```python
from build123d import *

# Parameters (mm, degrees)
SKETCH1_R           = 12.74408056
SKETCH1_R_2         = 4.1275
BOSS_EXTRUDE1_DEPTH = 6.35
SKETCH2_R           = 1.8415
CUT_EXTRUDE1_DEPTH  = 177.753707175


with BuildPart() as part:
    # Sketch1 → Boss-Extrude1 (new body)
    with BuildSketch(Plane(origin=(0, 0, 0), x_dir=(1, 0, 0), z_dir=(0, 1, 0))):
        with BuildLine():
            Line((0, -15.24), (158.75, -15.24))
            ThreePointArc((158.75, -15.24), (173.99, 0), (158.75, 15.24))
            Line((158.75, 15.24), (0, 15.24))
            ThreePointArc((0, 15.24), (-15.24, 0), (0, -15.24))
        make_face()
        with Locations(Location((0, 0, 0), (0, 0, 270))):
            Circle(SKETCH1_R, mode=Mode.SUBTRACT)
        with Locations(Location((31.75, 0, 0), (0, 0, 270))):
            Circle(SKETCH1_R, mode=Mode.SUBTRACT)
        with Locations(Location((63.5, 0, 0), (0, 0, 270))):
            Circle(SKETCH1_R, mode=Mode.SUBTRACT)
        with Locations(Location((95.25, 0, 0), (0, 0, 270))):
            Circle(SKETCH1_R, mode=Mode.SUBTRACT)
        with Locations(Location((127, 0, 0), (0, 0, 270))):
            Circle(SKETCH1_R, mode=Mode.SUBTRACT)
        with Locations(Location((158.75, 0, 0), (0, 0, 270))):
            Circle(SKETCH1_R, mode=Mode.SUBTRACT)
        with Locations(Location((15.875, -9.525, 0), (0, 0, 270))):
            Circle(SKETCH1_R_2, mode=Mode.SUBTRACT)
        with Locations(Location((15.875, 9.525, 0), (0, 0, 90))):
            Circle(SKETCH1_R_2, mode=Mode.SUBTRACT)
        with Locations(Location((79.375, 9.525, 0), (0, 0, 90))):
            Circle(SKETCH1_R_2, mode=Mode.SUBTRACT)
        with Locations(Location((79.375, -9.525, 0), (0, 0, 270))):
            Circle(SKETCH1_R_2, mode=Mode.SUBTRACT)
        with Locations(Location((142.875, 9.525, 0), (0, 0, 90))):
            Circle(SKETCH1_R_2, mode=Mode.SUBTRACT)
        with Locations(Location((142.875, -9.525, 0), (0, 0, 270))):
            Circle(SKETCH1_R_2, mode=Mode.SUBTRACT)
    extrude(amount=BOSS_EXTRUDE1_DEPTH)

    # Sketch2 → Cut-Extrude1 (cut, through all)
    with BuildSketch(Plane(origin=(0, 0, -15.24), x_dir=(-1, 0, 0), z_dir=(0, 0, -1))):
        with Locations((-111.125, 3.175)):
            Circle(SKETCH2_R)
        with Locations((-47.625, 3.175)):
            Circle(SKETCH2_R)
    extrude(amount=-CUT_EXTRUDE1_DEPTH, mode=Mode.SUBTRACT)


solid = part.part
```
Work out the finished part from the listing and answer in its coordinate system (mm). Round coordinates to 2 decimals unless told otherwise and drop trailing zeros. Order: outer loops, then holes, each group sorted by start corner. A loop starts at its lowest first (then second) coordinate and runs counter-clockwise, first axis right, second up.
Q1. A cutting plane is placed at A-A, the plane x = 95.25. Determine the outline of the cut face in (y, z).
Solution:
outline: (0, -15.24) - (6.35, -15.24) - (6.35, -12.74) - (0, -12.74) - close; (0, 12.74) - (6.35, 12.74) - (6.35, 15.24) - (0, 15.24) - close
Q2. A cutting plane is placed at C-C, the plane z = 9. Count the separate pieces of the cut face and the enclosed holes in it, then the cut area to 3 significant figures.
Solution:
separate pieces: 10
enclosed holes: 2
area: 299 mm2
Q3. Find the intervals of material crossed by line 1 along X through (y, z) = (3, -13); line 2 along Z through (x, y) = (141.5, 1); line 3 along X through (y, z) = (2.75, -13), in increasing order.
Solution:
line 1: x = -7.95 to 13.65, 18.1 to 45.79, 49.46 to 77.15, 81.6 to 109.29, 112.96 to 140.65, 145.1 to 166.7
line 2: z = -15.24 to -13.42, -5.63 to 5.63, 13.42 to 15.24
line 3: x = -7.95 to 13.65, 18.1 to 45.83, 49.42 to 77.15, 81.6 to 109.33, 112.92 to 140.65, 145.1 to 166.7
Q4. A cutting plane is placed at B-B, the plane x = 131. Determine the outline of the cut face in (y, z).
Solution:
outline: (0, -15.24) - (6.35, -15.24) - (6.35, -12.1) - (0, -12.1) - close; (0, 12.1) - (6.35, 12.1) - (6.35, 15.24) - (0, 15.24) - close
Q5. Given pin 1 Ø7.5 at (x, z) = (79.375, 9.525) entering from -Y; pin 2 Ø2 at (y, z) = (5.5, -3.5) entering from -X, each flat-ended and moving along its own axis, determine where each tip first touches the part or whether it passes through.
Solution:
pin 1: passes through
pin 2: stops at x = -15.03
Q6. The mould has two halves that part along Z. Classify faces 1 (the flat face through (80, 3, -15.24)), 2 (the cylindrical face through (75.283, 3.131, -8.988)), 3 (the flat face through (78, 3, 15.24)): pulls with the +Z half, pulls with the -Z half, needs draft (parallel to the pull), parting line crosses it, or undercut.
Solution:
face 1: pulls with the -Z half
face 2: undercut
face 3: pulls with the +Z half
